Answer from the drawing. Dimensions are ordinates in mm from the lowest x, y and z of the part. A direction names the side the tool comes from. Round coordinates to 2 decimals unless told otherwise and drop trailing zeros. Loops run counter-clockwise (first coordinate to the right, second up) from the corner with the lowest first, then second, coordinate; pieces in that order, holes last.
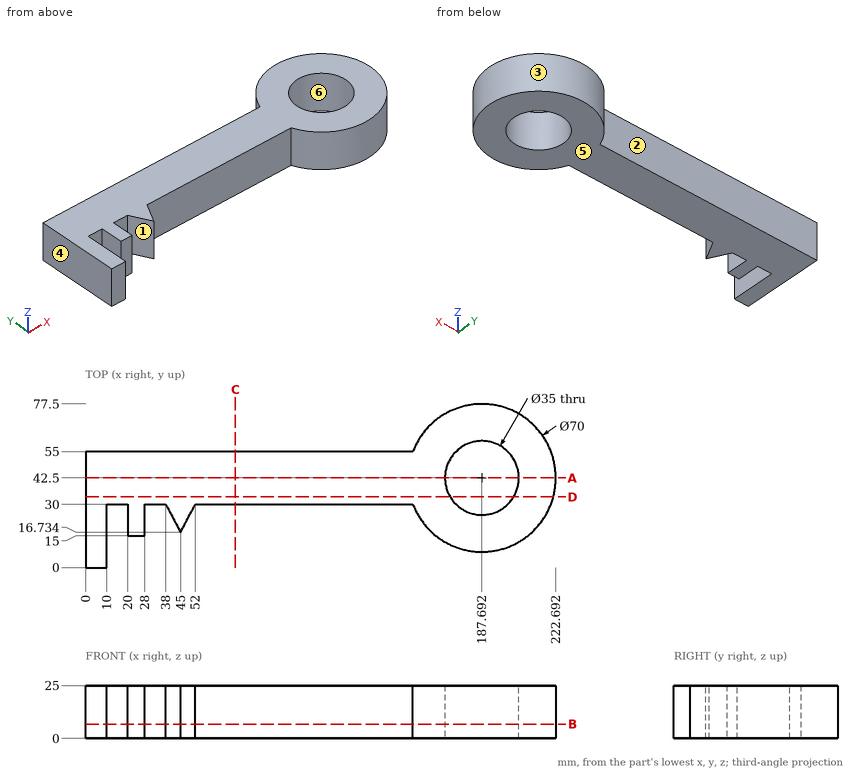
1. Determine the mould class of the marked faces 4, 5 and 6 for opening direction X: +X half, -X half, draft (parallel to the pull), parting line (faces both ways), or undercut.
Answer key:
face 4: -X half
face 5: draft
face 6: undercut
2. Find section D-D (y = 33.5). Write down the section's boundary in (x, z) (1 decimal), then the cut area to 3 significant figures.
Answer key:
outline: (0, 0) - (172.7, 0) - (172.7, 25) - (0, 25) - close; (202.7, 0) - (221.5, 0) - (221.5, 25) - (202.7, 25) - close
area: 4,790 mm2
3. Find section C-C (x = 71). Write down the section's boundary in (y, z).
Answer key:
outline: (30, 0) - (55, 0) - (55, 25) - (30, 25) - close
4. Which of the six approach directions +Z, -Z, +X, -X, +Y, -Y give full straight-line access (tool end or side, diameter ignored) to the marked faces 1, 2 and 3?
Answer key:
face 1: +Z, -Z, -Y
face 2: +Z, -Z, -X, +Y
face 3: +Z, -Z
5. Find section A-A (y = 42.5). Write down the section's boundary in (x, z), then the cut area to 3 significant figures.
Answer key:
outline: (0, 0) - (170.19, 0) - (170.19, 25) - (0, 25) - close; (205.19, 0) - (222.69, 0) - (222.69, 25) - (205.19, 25) - close
area: 4,690 mm2
6. Given pin 1 (8 mm diameter, centred on x = 182.5, z = 16, fed in from +Y); pin 2 (1 mm diameter, centred on x = 70.5, z = 7.5, fed in from -Y); pin 3 (2 mm diameter, centred on y = 23.5, z = 8, fed in from +X), each flat-ended and moving along its own axis, determine where each tip first touches the part or whether it passes through.
Answer key:
pin 1: stops at y = 77.48
pin 2: stops at y = 30
pin 3: stops at x = 217.71
7. Consider probe 1 along X at (y, z) = (36, 23.5) (1 decimal); probe 2 along Y at (x, z) = (83, 5.5); probe 3 along X at (y, z) = (37.5, 12). Determine where each line is inside the solid, lowest interval first.
Answer key:
probe 1: x = 0 to 171.4, 203.9 to 222.1
probe 2: y = 30 to 55
probe 3: x = 0 to 170.92, 204.46 to 222.33
8. Find section B-B (z = 6.75). Write down the section's boundary in (x, y).
Answer key:
outline: (0, 0) - (10, 0) - (10, 30) - (20, 30) - (20, 15) - (28, 15) - (28, 30) - (38, 30) - (45, 16.73) - (52, 30) - (155, 30) arc R35 ccw (long way) to (155, 55) - (0, 55) - close; hole circle Ø35 at (187.69, 42.5)
